Autodesk Inventor part; units mm, degrees
ref_plane "YZ Plane" through (0, 0, 0) normal (1, 0, 0) x (0, 1, 0)
ref_plane "XZ Plane" through (0, 0, 0) normal (0, 1, 0) x (-1, 0, 0)
ref_plane "XY Plane" through (0, 0, 0) normal (0, 0, 1) x (1, 0, 0)
sketch "Sketch1" plane through (0, 0, 0) normal (0, 1, 0) x (-1, 0, 0)
  line L0 (0, 0) -> (16, 0)
  line L1 (16, 0) -> (16, -12.3)
  line L2 (16, -12.3) -> (0, -12.3)
  line L3 (0, -12.3) -> (0, 0)
  dimension "d0" = 16
  dimension "d1" = 12.3
extrude "Extrusion1" add sketch "Sketch1" along normal blind 10
sketch "Sketch2" plane through (0, 10, 0) normal (0, 1, 0) x (1, 0, 0)
  line L0 (-16, 0) -> (0, 0)
  line L1 (-8, 0) -> (-8, 12.3)
  line L2 (0, 12.3) -> (-16, 12.3)
  line L3 (-14.5, 0) -> (-14.5, 12.3)
  line L4 (-1.5, 0) -> (-1.5, 12.3)
  dimension "d4" = 6.5
  dimension "d5" = 6.5
extrude "Extrusion2" add sketch "Sketch2" along normal blind 40.5
sketch "Sketch3" plane through (-16, 0, 0) normal (0, 0, 1) x (1, 0, 0)
  line L0 (14.5, 50.5) -> (1.5, 50.5)
  line L1 (8, 50.5) -> (8, 0)
  line L2 (0, 0) -> (16, 0)
  circle A0 centre (8, 44) radius 4.5
  line L3 (1.5, 50.5) -> (14.5, 50.5)
  circle A1 centre (8, 44) radius 6.5
  line L4 (14.5, 10) -> (14.5, 50.5)
  line L5 (14.5, 30.25) -> (1.5, 30.25)
  line L6 (1.5, 10) -> (1.5, 50.5)
  line L7 (8, 30.25) -> (11.5, 30.25)
  arc A2 (14.5, 44) -> (14.5, 10) centre (59.4062, 27) ccw
  line L8 (8, 30.25) -> (4.5, 30.25)
  arc A3 (1.5, 10) -> (1.5, 44) centre (-43.4062, 27) ccw
  dimension "d8" = 6.5
  dimension "d9" = 9
  dimension "d10" = 13
  dimension "d11" = 3.5
  dimension "d12" = 3.5
extrude "Extrusion3" cut sketch "Sketch3" against normal blind 13.5 contours L4 A1 L0 | A1 L6 L0 | L4 L5 A2 A1 | A1 A2 | A3 A1 | A1 A3 L5 L6 | L4 A2 L5 | L5 A3 L6
fillet "Fillet1" radius 10 4 edges at (0, 10, -6.15) (-1.5, 10, -6.15) (-14.5, 10, -6.15) (-16, 10, -6.15)
sketch "Sketch4" plane through (-16, 0, 0) normal (0, 0, 1) x (1, 0, 0)
  arc A0 (14.5, 44) -> (1.5, 44) centre (8, 44) ccw
  circle A1 centre (8, 44) radius 4.5
  point P0 (16, 0)
  dimension "d16" = 9
extrude "Extrusion4" cut sketch "Sketch4" against normal blind 8.23
sketch "Sketch5" plane through (0, 0, 0) normal (0, -1, 0) x (1, 0, 0)
  point P0 (0, 0)
sketch "Sketch7" plane through (-16, 0, 0) normal (0, 0, 1) x (1, 0, 0)
  line L0 (16, 0) -> (0, 0)
  line L1 (0, 0) -> (16, 0)
  line L2 (16, 0) -> (16, 10)
  line L3 (16, 10) -> (0, 10)
  line L4 (0, 10) -> (0, 0)
  line L5 (0, 5) -> (16, 5)
  line L6 (8, 10) -> (8, 0)
  circle A0 centre (4, 5) radius 1
  circle A1 centre (12, 5) radius 1
extrude "Extrusion6" cut sketch "Sketch7" against normal blind 12.3 contours A1 L5 | L5 A1 | A0 L5 | L5 A0
sketch "Sketch8" plane through (-16, 0, 0) normal (0, 0, 1) x (1, 0, 0)
  circle A0 centre (4, 5) radius 1
  circle A1 centre (4, 5) radius 2.25
  circle A2 centre (12, 5) radius 1
  circle A3 centre (12, 5) radius 2.25
  point P0 (16, 0)
  dimension "d24" = 4.5
  dimension "d25" = 4.5
extrude "Extrusion7" cut sketch "Sketch8" against normal blind 12.5
sketch "Sketch9" plane through (-16, 0, 0) normal (0, 0, 1) x (1, 0, 0)
  line L0 (0, 0) -> (0, 6.3517)
  line L1 (0, 5) -> (16, 5)
  point P0 (16, 0)
  point P1 (4, 5)
properties part number "pawn"
Work out the finished part from the listing and answer in its coordinate system (mm). A direction names the side the tool comes from. Coordinates: 2 decimals unless noted, no trailing zeros. Loops run counter-clockwise (first coordinate to the right, second up) from the corner with the lowest first, then second, coordinate; pieces in that order, holes last.
1) Flat-ended cylindrical pins translate along their axes: pin 1 (1 mm diameter, centred on x = -4.5, z = -2, fed in from +Y); pin 2 (5 mm diameter, centred on y = 14, z = -4, fed in from +X); pin 3 (2.5 mm diameter, centred on x = -9.5, y = 43.5, fed in from +Z); pin 4 (8 mm diameter, centred on x = -12, y = 34, fed in from -Z). Find the tip coordinate at first contact, or state that the pin passes through.
Results:
pin 1: stops at y = 49.77
pin 2: stops at x = -1.43
pin 3: stops at z = -8.23
pin 4: stops at z = -12.3
2) Section C-C (x = -8) is taken. Give the vertices of the cut face in (y, z).
Results:
outline: (0, -12.3) - (50.5, -12.3) - (50.5, 0) - (48.5, 0) - (48.5, -8.23) - (39.5, -8.23) - (39.5, 0) - (0, 0) - close
3) Section D-D (x = -5.25) is taken. Give the vertices of the cut face in (y, z).
Results:
outline: (0, -12.3) - (3.13, -12.3) - (3.13, 0) - (0, 0) - close; (6.87, -12.3) - (49.89, -12.3) - (49.89, 0) - (47.56, 0) - (47.56, -8.23) - (40.44, -8.23) - (40.44, 0) - (6.87, 0) - close
4) Section B-B (z = -6.5) is taken. Give the vertices of the cut face in (x, y).
Results:
outline: (-16, 0) - (0, 0) - (0, 6.35) arc R10 ccw to (-1.7, 11.94) arc R10 cw to (-3.09, 15.03) arc R48.02 cw to (-1.5, 44) arc R6.5 ccw to (-14.5, 44) arc R48.02 cw to (-12.91, 15.03) arc R10 cw to (-14.3, 11.94) arc R10 ccw to (-16, 6.35) - close; hole circle Ø4.5 at (-12, 5); hole circle Ø9 at (-8, 44); hole circle Ø4.5 at (-4, 5)
5) Consider probe 1 along Y at (x, z) = (-8.25, -5.5); probe 2 along X at (y, z) = (7, -6); probe 3 along Z at (x, y) = (-10, 47). Determine where each line is inside the solid, lowest interval first.
Results:
probe 1: y = 0 to 39.51, 48.49 to 50.5
probe 2: x = -15.98 to -13.03, -10.97 to -5.03, -2.97 to -0.02
probe 3: z = -12.3 to -8.23
6) For a pull along Y with two mould halves and no side action, classify faces 1 (the flat face through (-8, 25, -12.3)), 2 (the cylindrical face through (-4.526, 29.843, -6.064)), 3 (the flat face through (-8, 0, -6)) as +Y half, -Y half, draft (parallel to the pull), parting line (faces both ways), or undercut.
Results:
face 1: draft
face 2: undercut
face 3: -Y half
7) For faces 4 (the flat face through (-8, 44, -8.23)), 5 (the cylindrical face through (-7.9, 50.5, -6.1)), determine the directions among +Z, -Z, +X, -X, +Y, -Y from which every point of the face is accessible in a straight line to the end or side of a thin tool.
Results:
face 4: +Z
face 5: +Z, -Z, +Y
8) Section A-A (y = 5) is taken. Give the vertices of the cut face in (x, z), plus the area to 3 significant figures.
Results:
outline: (-16, -12.3) - (-14.25, -12.3) - (-14.25, 0) - (-16, 0) - close; (-9.75, -12.3) - (-6.25, -12.3) - (-6.25, 0) - (-9.75, 0) - close; (-1.75, -12.3) - (0, -12.3) - (0, 0) - (-1.75, 0) - close
area: 86.1 mm2
